The listing builds one solid part. Answer for the finished solid, in the listing's coordinates (mm). Face numbers are marked on the shaded views. A direction names the side the tool comes from. Give positions to 0.01 mm unless a question says otherwise; leave off trailing zeros. Order: outer loops, then holes, each group sorted by start corner. A loop starts at its lowest first (then second) coordinate and runs counter-clockwise, first axis right, second up. Notation, with made-up numbers: (11.25, 67) - (38.25, 67) arc R29 cw to (38.25, 88) - close; hole circle Ø2 at (-34, 61.25). An arc over 180 degrees is marked (long way). Use CSV: the item, a comma, the result in double quotes.
```python
from build123d import *

# Parameters (mm, degrees)
SKETCH1_W           = 71.12
SKETCH1_H           = 35.56
SKETCH1_R           = 1.905
SKETCH1_W_2         = 50.8
SKETCH1_H_2         = 20.32
BOSS_EXTRUDE1_DEPTH = 7.62
SKETCH3_W           = 35.56
SKETCH3_H           = 7.62
BOSS_EXTRUDE2_DEPTH = 12.7
SKETCH2_W           = 6.35
SKETCH2_H           = 2.032
SKETCH2_W_2         = 4.191
CUT_EXTRUDE1_DEPTH  = 61.428516447
FILLET1_R           = 3.175


with BuildPart() as part:
    # Sketch1 → Boss-Extrude1 (new body)
    with BuildSketch(Plane(origin=(0, 0, 0), x_dir=(1, 0, 0), z_dir=(0, 1, 0))):
        Rectangle(SKETCH1_W, SKETCH1_H)
        with Locations(Location((30.48, 12.7, 0), (0, 0, 90))):
            Circle(SKETCH1_R, mode=Mode.SUBTRACT)
        with Locations(Location((-30.48, 12.7, 0), (0, 0, 90))):
            Circle(SKETCH1_R, mode=Mode.SUBTRACT)
        with Locations(Location((-30.48, -12.7, 0), (0, 0, 90))):
            Circle(SKETCH1_R, mode=Mode.SUBTRACT)
        with Locations(Location((30.48, -12.7, 0), (0, 0, 90))):
            Circle(SKETCH1_R, mode=Mode.SUBTRACT)
        Rectangle(SKETCH1_W_2, SKETCH1_H_2, mode=Mode.SUBTRACT)
    extrude(amount=BOSS_EXTRUDE1_DEPTH)

    # Sketch3 → Boss-Extrude2 (add)
    with BuildSketch(Plane(origin=(35.56, 0, 0), x_dir=(0, 0, -1), z_dir=(1, 0, 0))):
        with Locations((0, 3.81)):
            Rectangle(SKETCH3_W, SKETCH3_H)
    extrude(amount=BOSS_EXTRUDE2_DEPTH)

    # Sketch2 → Cut-Extrude1 (cut, through all)
    with BuildSketch(Plane.XY.offset(17.78)):
        with BuildLine():
            Line((21.3995, 2.3495), (21.3995, 0))
            Line((21.3995, 0), (16.7005, 0))
            Line((16.7005, 0), (16.7005, 2.3495))
            ThreePointArc((16.7005, 2.3495), (19.05, 4.699), (21.3995, 2.3495))
        make_face()
        with BuildLine():
            Line((-2.0955, 2.3495), (-2.0955, 0))
            Line((-2.0955, 0), (-6.7945, 0))
            Line((-6.7945, 0), (-6.7945, 2.3495))
            ThreePointArc((-6.7945, 2.3495), (-4.445, 4.699), (-2.0955, 2.3495))
        make_face()
        with Locations((8.255, 1.016)):
            Rectangle(SKETCH2_W, SKETCH2_H)
        with Locations((-15.24, 1.016)):
            Rectangle(SKETCH2_W, SKETCH2_H)
        with BuildLine():
            Line((41.7195, 2.3495), (41.7195, 0))
            Line((41.7195, 0), (37.0205, 0))
            Line((37.0205, 0), (37.0205, 2.3495))
            ThreePointArc((37.0205, 2.3495), (39.37, 4.699), (41.7195, 2.3495))
        make_face()
        with Locations((-22.225, 1.016)):
            Rectangle(SKETCH2_W_2, SKETCH2_H)
    extrude(amount=-CUT_EXTRUDE1_DEPTH, mode=Mode.SUBTRACT)

    # Fillet1
    fillet1_edges = [part.edges().sort_by_distance(p)[0] for p in [
        (-35.56, 3.81, -17.78),
        (-35.56, 3.81, 17.78),
        (48.26, 3.81, -17.78),
        (48.26, 3.81, 17.78),
        (25.4, 3.81, 10.16),
        (25.4, 3.81, -10.16),
        (-25.4, 3.81, -10.16),
        (-25.4, 3.81, 10.16),
    ]]
    fillet(fillet1_edges, radius=FILLET1_R)


solid = part.part
```
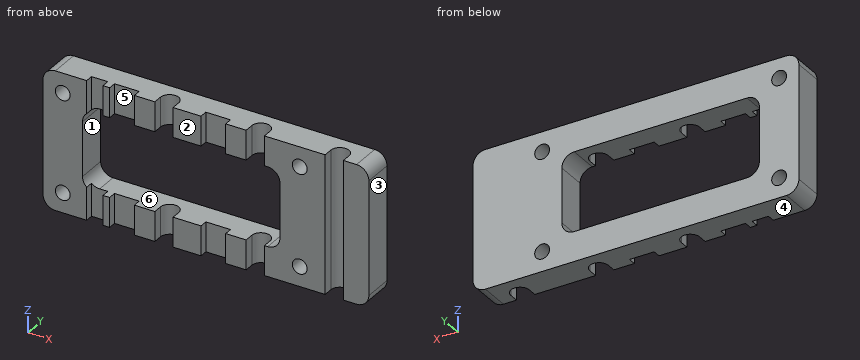
Item 1: The part is cut by section D-D (y = 6.75). Give the vertices of the cut face in (x, z) (3 decimals).
Taken from the geometry:
outline,"(-35.56, -14.605) arc R3.175 ccw to (-32.385, -17.78) - (45.085, -17.78) arc R3.175 ccw to (48.26, -14.605) - (48.26, 14.605) arc R3.175 ccw to (45.085, 17.78) - (-32.385, 17.78) arc R3.175 ccw to (-35.56, 14.605) - close; hole circle Ø3.81 at (-30.48, -12.7); hole circle Ø3.81 at (-30.48, 12.7); hole (-25.4, -6.985) arc R3.175 ccw to (-22.225, -10.16) - (22.225, -10.16) arc R3.175 ccw to (25.4, -6.985) - (25.4, 6.985) arc R3.175 ccw to (22.225, 10.16) - (-22.225, 10.16) arc R3.175 ccw to (-25.4, 6.985) - close; hole circle Ø3.81 at (30.48, -12.7); hole circle Ø3.81 at (30.48, 12.7)"
Item 2: Find the intervals of material crossed by line 1 along Z through (x, y) = (-30.48, 5) (3 decimals); line 2 along X through (y, z) = (2.25, 5); line 3 along X through (y, z) = (6, 12.7) (3 decimals), in increasing order.
Taken from the geometry:
line 1,"-17.78 to -14.605, -10.795 to 10.795, 14.605 to 17.78"
line 2,"-35.56 to -25.4, 25.4 to 37.02, 41.72 to 48.26"
line 3,"-35.56 to -32.385, -28.575 to 28.575, 32.385 to 48.26"
Item 3: The part is cut by section B-B (z = 6). Give the vertices of the cut face in (x, y).
Taken from the geometry:
outline,"(-35.56, 0) - (-25.4, 0) - (-25.4, 7.62) - (-35.56, 7.62) - close; (25.4, 0) - (37.02, 0) - (37.02, 2.35) arc R2.35 cw to (41.72, 2.35) - (41.72, 0) - (48.26, 0) - (48.26, 7.62) - (25.4, 7.62) - close"
Item 4: The mould has two halves that part along X. Classify the marked faces 1, 2 and 3: +X half, -X half, draft (parallel to the pull), parting line (faces both ways), or undercut.
Taken from the geometry:
face 1,"undercut"
face 2,"draft"
face 3,"+X half"
Item 5: Which of the six approach directions +Z, -Z, +X, -X, +Y, -Y give full straight-line access (tool end or side, diameter ignored) to the marked faces 4, 5 and 6?
Taken from the geometry:
face 4,"-Z, +X, -X, +Y, -Y"
face 5,"+Z, -Z, -Y"
face 6,"+Y, -Y"
Item 6: The part is cut by section C-C (x = -16.5). Give the vertices of the cut face in (y, z), and give its area (3 significant figures).
Taken from the geometry:
outline,"(2.03, -17.78) - (7.62, -17.78) - (7.62, -10.16) - (2.03, -10.16) - close; (2.03, 10.16) - (7.62, 10.16) - (7.62, 17.78) - (2.03, 17.78) - close"
area,"85.2 mm^2"
Item 7: The part is cut by section A-A (x = 30.48). Give the vertices of the cut face in (y, z) (3 decimals), and give its area (3 significant figures).
Taken from the geometry:
outline,"(0, -17.78) - (7.62, -17.78) - (7.62, -14.605) - (0, -14.605) - close; (0, -10.795) - (7.62, -10.795) - (7.62, 10.795) - (0, 10.795) - close; (0, 14.605) - (7.62, 14.605) - (7.62, 17.78) - (0, 17.78) - close"
area,"213 mm^2"
Item 8: This flat-tipped pin is pushed along its axis until it touches: pin 1 (3 mm diameter, centred on x = -16, z = 14.5, fed in from -Y). Where does it stop, or does it pass through?
Taken from the geometry:
pin 1,"y = 2.03"
